Work out the finished part from the listing and answer in its coordinate system (mm). A direction names the side the tool comes from. Round coordinates to 2 decimals unless told otherwise and drop trailing zeros. Order: outer loops, then holes, each group sorted by start corner. A loop starts at its lowest first (then second) coordinate and runs counter-clockwise, first axis right, second up. Notation, with made-up numbers: (62.5, -2.5) - (89.5, -2.5) arc R19 ccw to (89.5, 8.5) - close; hole circle Ø2 at (65.5, 13.25). An arc over 180 degrees is marked (long way). Use one line per item in the form item = value. Start each with the question number.
Q1. The part is cut by section C-C on z = -2.25. Determine the outline of the cut face in (x, y) (3 decimals), plus the area to 3 significant figures.
Q2. The part is cut by section A-A on z = 4.25. Determine the outline of the cut face in (x, y) (3 decimals), plus the area to 3 significant figures.
Q3. For a pull along Y with two mould halves and no side action, classify faces 5 (the flat face through (19.49, 0, 7)), 6 (the flat face through (0, 0, -3)), 7 (the flat face through (-16, 24.57, 7)) as +Y half, -Y half, draft (parallel to the pull), parting line (faces both ways), or undercut.
Q4. The part is cut by section D-D on y = 4. Determine the outline of the cut face in (x, z) (3 decimals), plus the area to 3 significant figures.
Q5. Given P1, Ø1, axis at x = 0, z = 7.5, coming from the +Y side; P2, Ø1.3, axis at x = -4.5, y = 24.5, coming from the +Z side; P3, Ø1, axis at x = 2, z = 6, coming from the +Y side (3 decimals), each flat-ended and moving along its own axis, determine where each tip first touches the part or whether it passes through.
Q6. Find the intervals of material crossed by line 1 (Y direction, x = -1.5, z = 0.5) (3 decimals); line 2 (X direction, y = 4, z = 1.25) (3 decimals); line 3 (Y direction, x = -18, z = 7) (3 decimals), in increasing order. Write a range as [from, to].
Q7. The part is cut by section B-B on x = 13. Determine the outline of the cut face in (y, z) (3 decimals), plus the area to 3 significant figures.
Q8. Which of the six approach directions +Z, -Z, +X, -X, +Y, -Y give full straight-line access (tool end or side, diameter ignored) to faces 1 (the flat face through (-19.49, 0, 7)), 2 (the flat face through (0, -24.57, 7)), 3 (the flat face through (-11.49, 25, 4)), 4 (the flat face through (0, 23.995, 1))?
from build123d import *

# Parameters (mm, degrees)
BOX029_W       = 10.25
BOX029_H       = 12
BOX029_DEPTH   = 13
BOX_W          = 10.25
BOX_H          = 12
BOX_DEPTH      = 13
BOX025_W       = 37.83
BOX025_H       = 47.99
BOX025_DEPTH   = 1.2
BOX026_W       = 38.98
BOX026_H       = 49.14
BOX026_DEPTH   = 1.2
BOX027_W       = 37.83
BOX027_H       = 47.99
BOX027_DEPTH   = 1.2
BOX028_W       = 40.25
BOX028_H       = 50.41
BOX028_DEPTH   = 1.2
BOX013_W       = 37.83
BOX013_H       = 47.99
BOX013_DEPTH   = 11
THICKNESS003_T = 1.2


with BuildPart() as cube029:
    # Box029 → Box029 (new body)
    with BuildSketch(Plane(origin=(-11.49, 14, 0.79), x_dir=(1, 0, 0), z_dir=(0, 0, 1))):
        with Locations((5.125, 6)):
            Rectangle(BOX029_W, BOX029_H)
    extrude(amount=BOX029_DEPTH)


with BuildPart() as cube:
    # Box → Box (new body)
    with BuildSketch(Plane(origin=(1.2, 14, 0.79), x_dir=(1, 0, 0), z_dir=(0, 0, 1))):
        with Locations((5.125, 6)):
            Rectangle(BOX_W, BOX_H)
    extrude(amount=BOX_DEPTH)


with BuildPart() as cube025:
    # Box025 → Box025 (new body)
    with BuildSketch(Plane(origin=(-18.91, -24, 0), x_dir=(1, 0, 0), z_dir=(0, 0, 1))):
        with Locations((18.915, 23.995)):
            Rectangle(BOX025_W, BOX025_H)
    extrude(amount=BOX025_DEPTH)


with BuildPart() as cut006:
    # Box026 → Box026 (new body)
    with BuildSketch(Plane(origin=(-19.49, -24.57, 0), x_dir=(1, 0, 0), z_dir=(0, 0, 1))):
        with Locations((19.49, 24.57)):
            Rectangle(BOX026_W, BOX026_H)
    extrude(amount=BOX026_DEPTH)

    # Cut006: cut Cube025
    add(cube025.part, mode=Mode.SUBTRACT)


with BuildPart() as cube027:
    # Box027 → Box027 (new body)
    with BuildSketch(Plane(origin=(-18.91, -24, 0), x_dir=(1, 0, 0), z_dir=(0, 0, 1))):
        with Locations((18.915, 23.995)):
            Rectangle(BOX027_W, BOX027_H)
    extrude(amount=BOX027_DEPTH)


with BuildPart() as cut008:
    # Box028 → Box028 (new body)
    with BuildSketch(Plane(origin=(-20.125, -25.205, 0), x_dir=(1, 0, 0), z_dir=(0, 0, 1))):
        with Locations((20.125, 25.205)):
            Rectangle(BOX028_W, BOX028_H)
    extrude(amount=BOX028_DEPTH)

    # Cut007: cut Cube027
    add(cube027.part, mode=Mode.SUBTRACT)

    # Cut008: cut Cut006
    add(cut006.part, mode=Mode.SUBTRACT)


with BuildPart() as cut008_1:
    # Cut008 placement: moved
    add(cut008.part.moved(Location((0, 0, 6.8))))


with BuildPart() as cut010:
    # Box013 → Box013 (new body)
    with BuildSketch(Plane(origin=(-18.915, -23.995, -3), x_dir=(1, 0, 0), z_dir=(0, 0, 1))):
        with Locations((18.915, 23.995)):
            Rectangle(BOX013_W, BOX013_H)
    extrude(amount=BOX013_DEPTH)


with BuildPart() as cut010_1:
    # BaseFeature001 placement: moved
    add(cut010.part.moved(Location((18.915, 23.995, 3))))

    # Thickness003
    thickness003_openings = [cut010_1.faces().sort_by_distance(p)[0] for p in [
        (18.915, 23.995, 11),
    ]]
    offset(amount=THICKNESS003_T, openings=thickness003_openings, kind=Kind.INTERSECTION)


with BuildPart() as cut010_2:
    # Body001 placement: moved
    add(cut010_1.part.moved(Location((-18.915, -23.995, -3))))

    # Cut: cut Cut008
    add(cut008_1.part, mode=Mode.SUBTRACT)

    # Cut009: cut Cube
    add(cube.part, mode=Mode.SUBTRACT)

    # Cut010: cut Cube029
    add(cube029.part, mode=Mode.SUBTRACT)


solid = cut010_2.part
Found:
q1.outline = (-20.115, -25.195) - (20.115, -25.195) - (20.115, 25.195) - (-20.115, 25.195) - close; hole (-18.915, -23.995) - (18.915, -23.995) - (18.915, 23.995) - (-18.915, 23.995) - close
q1.area = 212 mm²
q2.outline = (-20.115, -25.195) - (20.115, -25.195) - (20.115, 25.195) - (11.45, 25.195) - (11.45, 23.995) - (18.915, 23.995) - (18.915, -23.995) - (-18.915, -23.995) - (-18.915, 23.995) - (-11.49, 23.995) - (-11.49, 25.195) - (-20.115, 25.195) - close; (-1.24, 23.995) - (1.2, 23.995) - (1.2, 25.195) - (-1.24, 25.195) - close
q2.area = 187 mm²
q3.face_5 = draft
q3.face_6 = undercut
q3.face_7 = +Y half
q4.outline = (-20.115, -4.2) - (20.115, -4.2) - (20.115, 6.8) - (19.49, 6.8) - (19.49, 8) - (18.915, 8) - (18.915, -3) - (-18.915, -3) - (-18.915, 8) - (-19.49, 8) - (-19.49, 6.8) - (-20.115, 6.8) - close
q4.area = 73.2 mm²
q5.P1 = 24.57
q5.P2 = 0.79
q5.P3 = -23.995
q6.line_1 = [-25.195, -23.995], [23.995, 25.195]
q6.line_2 = [-20.115, -18.915], [18.915, 20.115]
q6.line_3 = [-24.57, -23.995], [23.995, 24.57]
q7.outline = (-25.195, -4.2) - (25.195, -4.2) - (25.195, 6.8) - (24.57, 6.8) - (24.57, 8) - (23.995, 8) - (23.995, -3) - (-23.995, -3) - (-23.995, 8) - (-24.57, 8) - (-24.57, 6.8) - (-25.195, 6.8) - close
q7.area = 85.4 mm²
q8.face_1 = +Z, -X, +Y, -Y
q8.face_2 = +Z, +X, -X, -Y
q8.face_3 = +Z, +Y
q8.face_4 = +Z
